Here's the drawing with two shaded views (mm, measured from the low corner). I have some questions. Give positions to 0.01 mm unless a question says otherwise; leave off trailing zeros. Loops run counter-clockwise (first coordinate to the right, second up) from the corner with the lowest first, then second, coordinate; pieces in that order, holes last. Notation, with made-up numbers: (79.25, 60) - (91.25, 60) arc R22 cw to (91.25, 90) - close; hole circle Ø6 at (47.5, 85). An arc over 180 degrees is marked (long way). Write each question's results on one line, items separated by ' | '. Start each with the question number.
1) I want a section at C-C, the plane x = 29.5. Write out the boundary of the cut face in (y, z).
2) If we mould it in two halves opening along X, with no side actions, what happens to the marked faces 1, 2 and 3? For each: +X half, -X half, draft (parallel to the pull), parting line (faces both ways), or undercut.
3) I want a section at A-A, the plane z = 29.5. Write out the boundary of the cut face in (x, y).
4) If I drill on probe 1 along X at (y, z) = (3.7, 29.5); probe 2 along Z at (x, y) = (39, 3.5); probe 3 along Y at (x, z) = (26, 54), over which ranges is the centre line in solid material (lowest first)? Write a range as [from, to].
5) I'm going to push flat-ended pins straight in: pin 1 (6 mm diameter, centred on x = 39.5, y = 6, fed in from -Z) (3 decimals); pin 2 (5 mm diameter, centred on y = 5.5, z = 42.5, fed in from -X); pin 3 (8 mm diameter, centred on x = 38, z = 47.5, fed in from +Y). Where does each tip first touch, or does it pass through?
6) I want a section at D-D, the plane y = 4. Write out the boundary of the cut face in (x, z) (3 decimals).
7) I want a section at B-B, the plane x = 45.5. Write out the boundary of the cut face in (y, z), and give its area (3 significant figures).
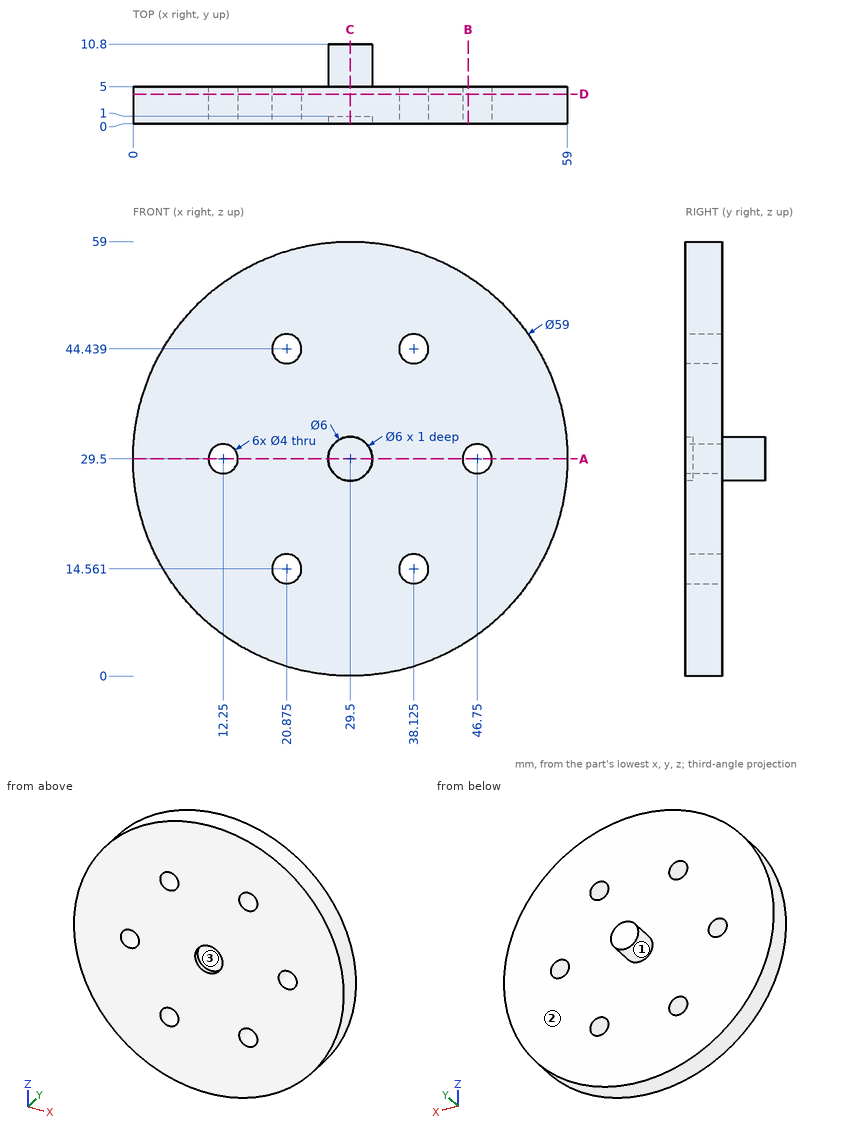
Answers:
1) outline: (0, 0) - (5, 0) - (5, 26.5) - (10.8, 26.5) - (10.8, 32.5) - (5, 32.5) - (5, 59) - (0, 59) - (0, 32.5) - (1, 32.5) - (1, 26.5) - (0, 26.5) - close
2) face 1: parting line | face 2: draft | face 3: undercut
3) outline: (0, 0) - (10.25, 0) - (10.25, 5) - (0, 5) - close; (14.25, 0) - (26.5, 0) - (26.5, 1) - (32.5, 1) - (32.5, 0) - (44.75, 0) - (44.75, 5) - (32.5, 5) - (32.5, 10.8) - (26.5, 10.8) - (26.5, 5) - (14.25, 5) - close; (48.75, 0) - (59, 0) - (59, 5) - (48.75, 5) - close
4) probe 1: x = [0, 10.25], [14.25, 44.75], [48.75, 59] | probe 2: z = [1.57, 12.76], [16.36, 42.64], [46.24, 57.43] | probe 3: y = [0, 5]
5) pin 1: stops at z = 0.885 | pin 2: stops at x = 1.95 | pin 3: stops at y = 5
6) outline: circle Ø59 at (29.5, 29.5); hole circle Ø4 at (12.25, 29.5); hole circle Ø4 at (20.875, 14.561); hole circle Ø4 at (20.875, 44.439); hole circle Ø4 at (38.125, 14.561); hole circle Ø4 at (38.125, 44.439); hole circle Ø4 at (46.75, 29.5)
7) outline: (0, 4.72) - (5, 4.72) - (5, 27.94) - (0, 27.94) - close; (0, 31.06) - (5, 31.06) - (5, 54.28) - (0, 54.28) - close | area: 232 mm2
